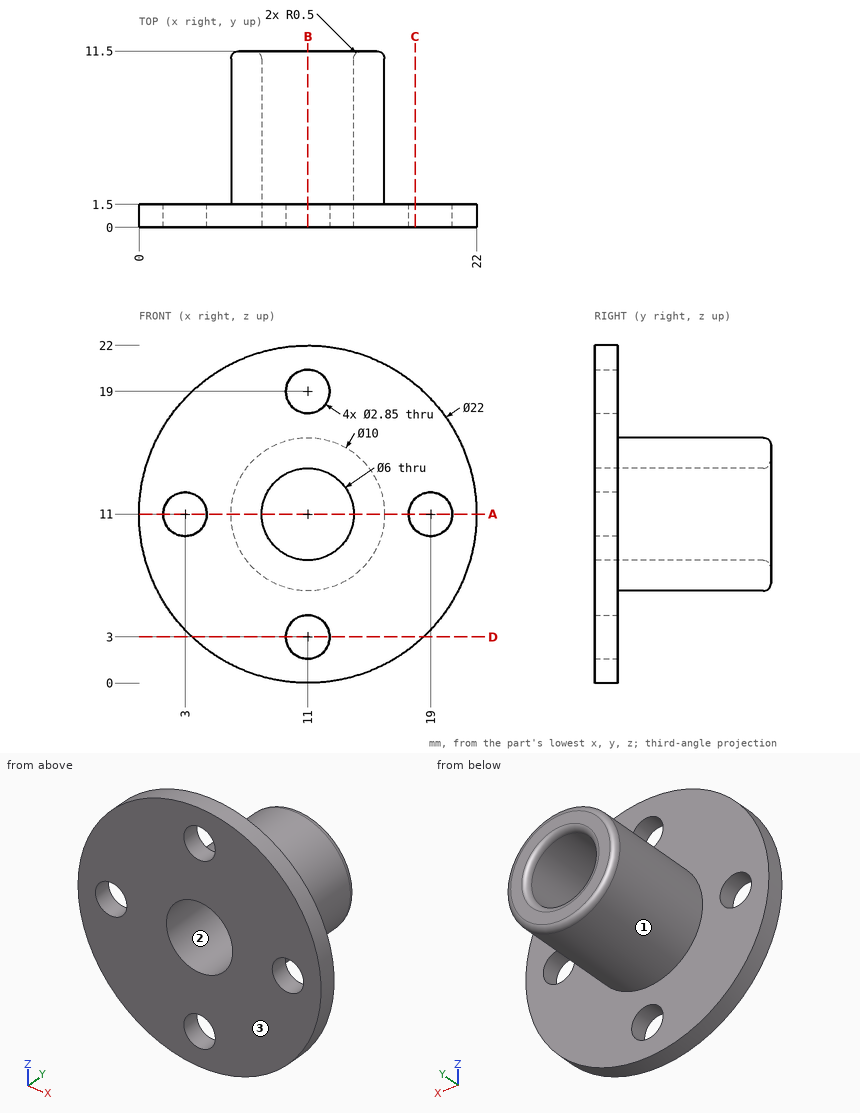
Verification items for this drawing (mm, ordinates from the low corner). Coordinates: 2 decimals unless noted, no trailing zeros. Order: outer loops, then holes, each group sorted by start corner. A loop starts at its lowest first (then second) coordinate and runs counter-clockwise, first axis right, second up. Notation, with made-up numbers: (8.5, 35.25) - (64.5, 35.25) arc R11 ccw to (64.5, 41.25) - close; hole circle Ø8 at (49, -32.5). An arc over 180 degrees is marked (long way). Answer as a JSON object with one key per item and string values. Group by question number.
Item 1: Sectioned sample at C-C, the plane x = 18. Record the cut outline in (y, z).
Item 2: Sectioned sample at B-B, the plane x = 11. Record the cut outline in (y, z) (3 decimals).
Item 3: Scan lines: probe 1 along Z at (x, y) = (11, 5.5); probe 2 along Y at (x, z) = (15.5, 18.25); probe 3 along Z at (x, y) = (19, 0.5) (3 decimals). Record each from-to range of solid material in increasing order.
Item 4: Draft check along Z on the marked faces 1, 2 and 3. Enter one of: +Z half, -Z half, draft (parallel to the pull), parting line (faces both ways), or undercut.
Item 5: Sectioned sample at D-D, the plane z = 3. Record the cut outline in (x, y) (3 decimals), and give its area (3 significant figures).
Item 6: Sectioned sample at A-A, the plane z = 11. Record the cut outline in (x, y) (3 decimals).
Item 7: Depth check by flat-ended pin: pin 1 Ø4.5 at (x, z) = (3, 11) entering from +Y; pin 2 Ø2 at (x, z) = (14, 16) entering from +Y; pin 3 Ø6 at (y, z) = (8.5, 6) entering from -X. Enter the tip coordinate at first touch or a pass-through.
Resolved:
{
 "1": {"outline": "(0, 2.51) - (1.5, 2.51) - (1.5, 9.98) - (0, 9.98) - close; (0, 12.02) - (1.5, 12.02) - (1.5, 19.49) - (0, 19.49) - close"},
 "2": {"outline": "(0, 0) - (1.5, 0) - (1.5, 1.575) - (0, 1.575) - close; (0, 4.425) - (1.5, 4.425) - (1.5, 6) - (11, 6) arc R0.5 ccw to (11.5, 6.5) - (11.5, 7.5) arc R0.5 ccw to (11, 8) - (0, 8) - close; (0, 14) - (11, 14) arc R0.5 ccw to (11.5, 14.5) - (11.5, 15.5) arc R0.5 ccw to (11, 16) - (1.5, 16) - (1.5, 17.575) - (0, 17.575) - close; (0, 20.425) - (1.5, 20.425) - (1.5, 22) - (0, 22) - close"},
 "3": {"probe 1": "6 to 8, 14 to 16", "probe 2": "0 to 1.5", "probe 3": "3.45 to 9.575, 12.425 to 18.55"},
 "4": {"face 1": "parting line", "face 2": "undercut", "face 3": "draft"},
 "5": {"outline": "(3.45, 0) - (9.575, 0) - (9.575, 1.5) - (3.45, 1.5) - close; (12.425, 0) - (18.55, 0) - (18.55, 1.5) - (12.425, 1.5) - close", "area": "18.4 mm^2"},
 "6": {"outline": "(0, 0) - (1.575, 0) - (1.575, 1.5) - (0, 1.5) - close; (4.425, 0) - (8, 0) - (8, 11) arc R0.5 ccw to (7.5, 11.5) - (6.5, 11.5) arc R0.5 ccw to (6, 11) - (6, 1.5) - (4.425, 1.5) - close; (14, 0) - (17.575, 0) - (17.575, 1.5) - (16, 1.5) - (16, 11) arc R0.5 ccw to (15.5, 11.5) - (14.5, 11.5) arc R0.5 ccw to (14, 11) - close; (20.425, 0) - (22, 0) - (22, 1.5) - (20.425, 1.5) - close"},
 "7": {"pin 1": "y = 1.5", "pin 2": "y = 11.37", "pin 3": "x = 6.42"}
}
